For this review, take the finished solid that the model builds, in its own axes (mm). A direction names the side the tool comes from. Give positions to 0.01 mm unless a question says otherwise; leave off trailing zeros. Order: outer loops, then holes, each group sorted by start corner. A loop starts at its lowest first (then second) coordinate and runs counter-clockwise, first axis right, second up.
from build123d import *

# Parameters (mm, degrees)
SKETCH1_R           = 9.525
SKETCH1_R_2         = 3.25
BOSS_EXTRUDE1_DEPTH = 20
SKETCH2_R           = 11
BOSS_EXTRUDE2_DEPTH = 7
SKETCH3_R           = 3.27
CUT_EXTRUDE1_DEPTH  = 7


with BuildPart() as part:
    # Sketch1 → Boss-Extrude1 (new body)
    with BuildSketch(Plane.XY):
        Circle(SKETCH1_R)
        Circle(SKETCH1_R_2, mode=Mode.SUBTRACT)
    extrude(amount=BOSS_EXTRUDE1_DEPTH)

    # Sketch2 → Boss-Extrude2 (add)
    with BuildSketch(Plane.XY.offset(20)):
        with Locations(Location((0, 0, 0), (0, 0, 180))):
            Circle(SKETCH2_R)
    extrude(amount=BOSS_EXTRUDE2_DEPTH)

    # Sketch3 → Cut-Extrude1 (cut)
    with BuildSketch(Plane.XY.offset(27)):
        Circle(SKETCH3_R)
    extrude(amount=-CUT_EXTRUDE1_DEPTH, mode=Mode.SUBTRACT)


solid = part.part
1) We need section A-A on y = 0. Give the boundary of the cut face in (x, z) (3 decimals), then the cut area to 3 significant figures.
Answer sheet:
outline: (-11, 20) - (-9.525, 20) - (-9.525, 0) - (-3.25, 0) - (-3.25, 20) - (-3.27, 20) - (-3.27, 27) - (-11, 27) - close; (3.25, 0) - (9.525, 0) - (9.525, 20) - (11, 20) - (11, 27) - (3.27, 27) - (3.27, 20) - (3.25, 20) - close
area: 359 mm2
2) Clearance check with flat-ended pins moving along their axes: pin 1 (5 mm diameter, centred on x = -7, z = 14.5, fed in from +Y) (3 decimals); pin 2 (1 mm diameter, centred on x = 6.5, z = 13.5, fed in from -Y); pin 3 (12 mm diameter, centred on y = -5, z = 12, fed in from +X) (3 decimals); pin 4 (2 mm diameter, centred on x = -1, y = -1, fed in from +Z) (3 decimals). State where each tip first meets the part, or that it passes through.
Answer sheet:
pin 1: stops at y = 8.395
pin 2: stops at y = -7.4
pin 3: stops at x = 9.525
pin 4: passes through
3) Draft analysis for pull direction X (two halves, no side actions). For faces 1 (the face through (0, -10, 20)), 2 (the face through (3.12, 0.98, 23.55)), 3 (the face through (-2.579, -1.978, 9.86)), 4 (the face through (2.38, 10.74, 23.45)), state which applies: +X half, -X half, draft (parallel to the pull), parting line (faces both ways), or undercut.
Answer sheet:
face 1: draft
face 2: undercut
face 3: undercut
face 4: parting line
4) To check wall thickness, follow line 1 (Y direction, x = 0, z = 23); line 2 (X direction, y = -1.5, z = 14.25); line 3 (Z direction, x = 9.25, y = -5). State the ranges of each line that lie inside material, in increasing order.
Answer sheet:
line 1: y = -11 to -3.27, 3.27 to 11
line 2: x = -9.41 to -2.88, 2.88 to 9.41
line 3: z = 20 to 27
5) Tool access review of faces 5 (the face through (-7.559, -5.796, 9.86)), 6 (the face through (3, 2, 27)): name each direction out of +Z, -Z, +X, -X, +Y, -Y from which nothing blocks a thin tool from reaching the whole face with its end or side.
Answer sheet:
face 5: -Z
face 6: +Z, +X, -X, +Y, -Y
6) We need section C-C on z = 3.75. Give the boundary of the cut face in (x, y) (3 decimals).
Answer sheet:
outline: circle Ø19.05 at (0, 0); hole circle Ø6.5 at (0, 0)
7) We need section D-D on x = -6.25. Give the boundary of the cut face in (y, z).
Answer sheet:
outline: (-9.05, 20) - (-7.19, 20) - (-7.19, 0) - (7.19, 0) - (7.19, 20) - (9.05, 20) - (9.05, 27) - (-9.05, 27) - close
